Here's how the part is built. I have some questions about the finished solid (model axes, mm). A direction names the side the tool comes from. Coordinates: 2 decimals unless noted, no trailing zeros. Write each loop counter-clockwise with the first axis right and the second up, starting at its lowest first coordinate (ties: lowest second). Pieces come first, ordered by that corner, then holes. Notation, with made-up numbers: M -39.75,42.25 L -26.75,42.25 A28 ccw -26.75,60.25 Z; hole C 33.5,63 d10. An arc over 180 degrees is marked long. Use a Markdown table: item, result.
Autodesk Inventor part; units mm, degrees
ref_plane "YZ Plane" through (0, 0, 0) normal (1, 0, 0) x (0, 1, 0)
ref_plane "XZ Plane" through (0, 0, 0) normal (0, 1, 0) x (-1, 0, 0)
ref_plane "XY Plane" through (0, 0, 0) normal (0, 0, 1) x (1, 0, 0)
sketch "Sketch1" plane through (0, 0, 0) normal (0, 1, 0) x (-1, 0, 0)
  circle A0 centre (0, 0) radius 4
  line L0 (0, 0) -> (0, -28) construction
  line L1 (-15, -29) -> (15, -29)
  line L2 (15, -29) -> (15, -27)
  line L3 (15, -27) -> (-15, -27)
  line L4 (-15, -27) -> (-15, -29)
  line L5 (-15, -29) -> (15, -27) construction
  line L6 (15, -29) -> (-15, -27) construction
  circle A1 centre (0, 0) radius 7
  line L7 (0, -7) -> (0, -27)
  line L8 (-7, 0) -> (-7, -27)
  dimension "d0" = 8
  dimension "d1" = 28
  dimension "d2" = 30
  dimension "d3" = 2
  dimension "d4" = 3
extrude "Extrusion1" add sketch "Sketch1" along normal blind 10
sketch "Sketch2" plane through (0, 10, 0) normal (0, 1, 0) x (1, 0, 0)
  line L0 (15, 29) -> (-15, 29)
  line L1 (7, 27) -> (15, 27)
  line L2 (-15, 29) -> (15, 29)
  line L3 (15, 29) -> (15, 27)
  line L4 (15, 27) -> (-15, 27)
  line L5 (-15, 27) -> (-15, 29)
  point P0 (0, 0)
extrude "Extrusion2" add sketch "Sketch2" along normal blind 20
fillet "Fillet1" radius 10 3 edges at (7, 5, -27) (0, 5, -27) (0, 5, -7)
properties part number "pivotholder"
1. Which directions (+Z, -Z, +X, -X, +Y, -Y) give clear straight access to the entire face, cutting with the end or side of a thin tool? Please do faces 5 (the face through (7, 5, -8)), 6 (the face through (-1.06, 4.93, -9.27)), 7 (the face through (0, 30, -28)).
Answers follow:
| item | result |
|---|---|
| face 5 | +Z, +X, +Y, -Y |
| face 6 | -X, +Y, -Y |
| face 7 | +Z, -Z, +X, -X, +Y |
2. Suppose I cut it at C-C on x = 0.5. Write out the boundary of the cut face in (y, z), and give its area (3 significant figures).
Answers follow:
| item | result |
|---|---|
| outline | M 0,-29 L 30,-29 L 30,-27 L 10,-27 L 10,-3.97 L 0,-3.97 Z; M 0,3.97 L 10,3.97 L 10,6.98 L 0,6.98 Z |
| area | 320 mm2 |
3. Suppose I cut it at A-A on y = 3. Write out the boundary of the cut face in (x, z), and give its area (3 significant figures).
Answers follow:
| item | result |
|---|---|
| outline | M -15,-29 L 15,-29 L 15,-27 A10 cw 7,-17.2 L 7,0 A7 ccw long -4.12,-5.66 A10 cw 0,-13.75 L 0,-17 A10 cw -10,-27 L -15,-27 Z; hole C 0,0 d8 |
| area | 362 mm2 |
4. Will these pins go through, and if not, where does the flat tip stop? pin 1 Ø5 at (y, z) = (7, -11.5) entering from +X; pin 2 Ø8 at (y, z) = (10.5, 2) entering from -X; pin 3 Ø2 at (x, z) = (2.5, 3.5) entering from +Y.
Answers follow:
| item | result |
|---|---|
| pin 1 | stops at x = 7 |
| pin 2 | stops at x = -7 |
| pin 3 | stops at y = 10 |
5. I need wall thicknesses on probe 1 along Y at (x, z) = (13, -26.5); probe 2 along X at (y, z) = (4.5, -1.5); probe 3 along Z at (x, y) = (-5.25, 1.75). Which ranges of each line are inside material? Lowest first, please.
Answers follow:
| item | result |
|---|---|
| probe 1 | y = 0 to 10 |
| probe 2 | x = -6.84 to -3.71, 3.71 to 7 |
| probe 3 | z = -29 to -25.8, -4.63 to 4.63 |
6. Suppose I cut it at D-D on x = -3.5. Write out the boundary of the cut face in (y, z), and give its area (3 significant figures).
Answers follow:
| item | result |
|---|---|
| outline | M 0,-29 L 30,-29 L 30,-27 L 10,-27 L 10,-24.6 L 0,-24.6 Z; M 0,-6.15 L 10,-6.15 L 10,-1.94 L 0,-1.94 Z; M 0,1.94 L 10,1.94 L 10,6.06 L 0,6.06 Z |
| area | 167 mm2 |
7. We'd pull the mould along Z, two halves only. Please class faces 1 (the face through (0, 18, -27)), 2 (the face through (-3.01, 4.93, -24.15)), 3 (the face through (2, 10, -11)), 4 (the face through (0.867, 4.93, 3.905)): +Z half, -Z half, draft (parallel to the pull), parting line (faces both ways), or undercut.
Answers follow:
| item | result |
|---|---|
| face 1 | +Z half |
| face 2 | undercut |
| face 3 | draft |
| face 4 | undercut |
8. Suppose I cut it at B-B on z = 2. Write out the boundary of the cut face in (x, y).
Answers follow:
| item | result |
|---|---|
| outline | M -6.71,0 L -3.46,0 L -3.46,10 L -6.71,10 Z; M 3.46,0 L 6.71,0 L 6.71,10 L 3.46,10 Z |
